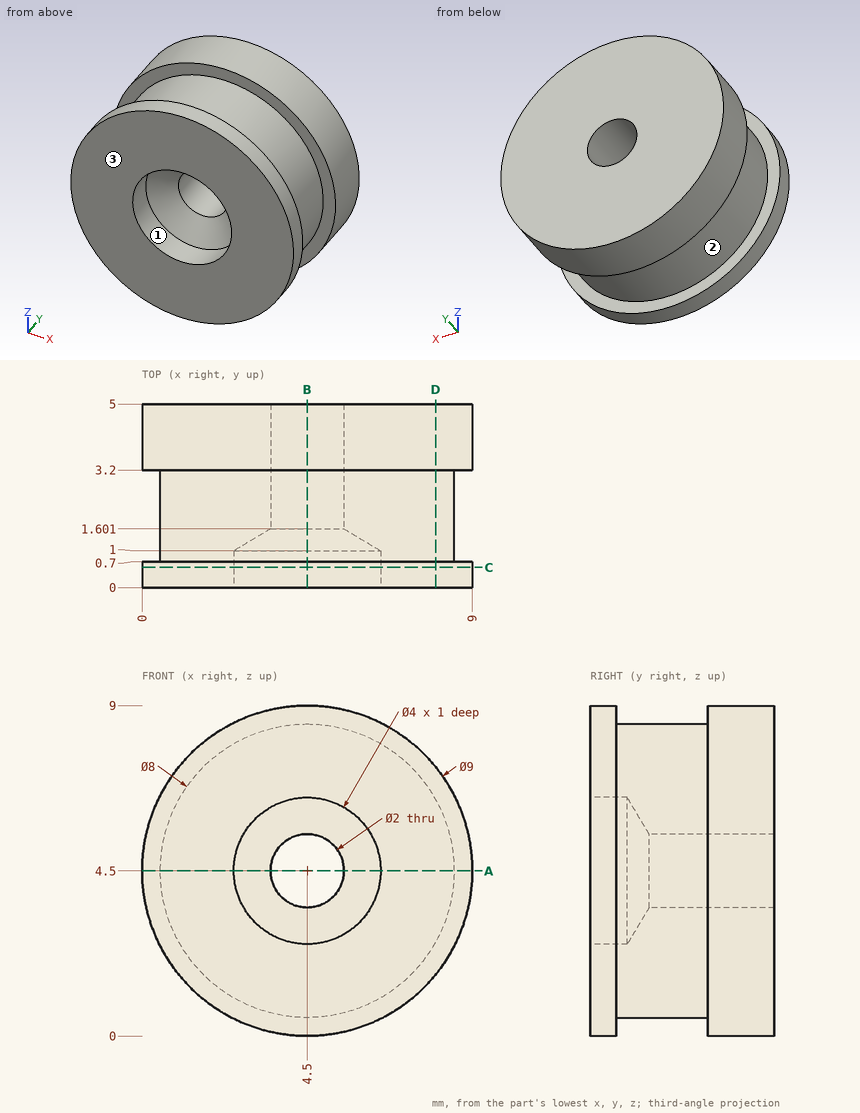
Source: three-view drawing plus pictorial views. Frame: mm from the lowest corner of the part. Round coordinates to 2 decimals unless told otherwise and drop trailing zeros. Order: outer loops, then holes, each group sorted by start corner. A loop starts at its lowest first (then second) coordinate and runs counter-clockwise, first axis right, second up. Notation, with made-up numbers: (69.25, -31) -> (112.25, -31) arc R28 ccw to (112.25, 6) -> close; hole circle Ø11 at (35.5, -8.75). An arc over 180 degrees is marked (long way). Use one line per item in the form item = value.
(1) Section D-D on x = 8. Return loops of the section in (y, z).
Results list:
outline = (0, 1.67) -> (0.7, 1.67) -> (0.7, 2.56) -> (3.2, 2.56) -> (3.2, 1.67) -> (5, 1.67) -> (5, 7.33) -> (3.2, 7.33) -> (3.2, 6.44) -> (0.7, 6.44) -> (0.7, 7.33) -> (0, 7.33) -> close
(2) First-contact query: pin 1 Ø1 at (y, z) = (3, 5.5) entering from +X; pin 2 Ø1.5 at (x, y) = (4.5, 1.5) entering from -Z; pin 3 Ø3 at (x, y) = (3, 4) entering from +Z. Flat tips, straight axial feed; report the tip coordinate or a pass-through.
Results list:
pin_1 = 8.97
pin_2 = 0.5
pin_3 = 9
(3) Draft query along X for the marked faces 1, 2 and 3. Return one class per face: pulls with the +X half, pulls with the -X half, needs draft (parallel to the pull), parting line crosses it, or undercut.
Results list:
face_1 = undercut
face_2 = parting line crosses it
face_3 = needs draft
(4) Ray query, probe 1 along X at (y, z) = (3.8, 4.5); probe 2 along X at (y, z) = (2.35, 4.5); probe 3 along Y at (x, z) = (7.25, 7.5). Return the intervals inside material, ascending. Write a range as [from, to].
Results list:
probe_1 = [0, 3.5], [5.5, 9]
probe_2 = [0.5, 3.5], [5.5, 8.5]
probe_3 = [0, 0.7], [3.2, 5]
(5) Section A-A on z = 4.5. Return loops of the section in (x, y).
Results list:
outline = (0, 0) -> (2.5, 0) -> (2.5, 1) -> (3.5, 1.6) -> (3.5, 5) -> (0, 5) -> (0, 3.2) -> (0.5, 3.2) -> (0.5, 0.7) -> (0, 0.7) -> close; (5.5, 1.6) -> (6.5, 1) -> (6.5, 0) -> (9, 0) -> (9, 0.7) -> (8.5, 0.7) -> (8.5, 3.2) -> (9, 3.2) -> (9, 5) -> (5.5, 5) -> close
(6) Section C-C on y = 0.55. Return loops of the section in (x, z).
Results list:
outline = circle Ø9 at (4.5, 4.5); hole circle Ø4 at (4.5, 4.5)
(7) Section B-B on x = 4.5. Return loops of the section in (y, z).
Results list:
outline = (0, 0) -> (0.7, 0) -> (0.7, 0.5) -> (3.2, 0.5) -> (3.2, 0) -> (5, 0) -> (5, 3.5) -> (1.6, 3.5) -> (1, 2.5) -> (0, 2.5) -> close; (0, 6.5) -> (1, 6.5) -> (1.6, 5.5) -> (5, 5.5) -> (5, 9) -> (3.2, 9) -> (3.2, 8.5) -> (0.7, 8.5) -> (0.7, 9) -> (0, 9) -> close
